Build history of the part. All positions in model axes, mm. Coordinates: 2 decimals unless noted, no trailing zeros. Order: outer loops, then holes, each group sorted by start corner. A loop starts at its lowest first (then second) coordinate and runs counter-clockwise, first axis right, second up. Notation, with made-up numbers: M 12.25,21.5 L 54.25,21.5 A7 ccw 54.25,33.5 Z; hole C 25,25.25 d7. An arc over 180 degrees is marked long. Write item = value, one per line. Start each with the question number.
Q1. Band-saw the part on B-B on x = 95.5. Write the cut outline in (y, z), plus the area to 3 significant figures.
Q2. Band-saw the part on A-A on z = 9.5. Write the cut outline in (x, y).
Q3. Band-saw the part on D-D on x = 34.5. Write the cut outline in (y, z).
Q4. Band-saw the part on C-C on y = -631.5. Write the cut outline in (x, z).
Q5. Drill centre lines: probe 1 along Z at (x, y) = (65, -531); probe 2 along Y at (x, z) = (293, 19.5); probe 3 along Y at (x, z) = (161.5, 29). Where is each one in solid material? Low to high.
Q6. Pin check, flat tips, straight feed: P1, Ø1.1, axis at x = 155, z = -0.5, coming from the +Y side; P2, Ø6, axis at x = 193.5, y = -675, coming from the -Z side; P3, Ø20, axis at x = 293, y = -1080.5, coming from the +Z side; P4, Ø6.5, axis at y = -1114.5, z = 7.5, coming from the +X side. Stop position of each tip, or through.
Q7. Pull direction Z, two halves, no side cores. Call faces 1 (the face through (299, -1083, 20.9)), 2 (the face through (184.49, -576.194, 9.853)), 3 (the face through (162, -606, 41.5)), 4 (the face through (196.1, -567.9, 14.2)): released by +Z, released by -Z, zero draft, split by the parting line, or undercut.
```python
from build123d import *

# Parameters (mm, degrees)
SKETCH_1_W        = 15.2
SKETCH_1_H        = 25
SKETCH_1_W_2      = 15.9
SKETCH_1_W_3      = 60
SKETCH_1_H_2      = 55.8
SKETCH_1_H_3      = 56.6
SKETCH_1_H_4      = 59.4
SKETCH_1_W_4      = 147.9
SKETCH_1_H_5      = 26.5
SKETCH_1_H_6      = 78.6
SKETCH_1_H_7      = 80.6
SKETCH_1_H_8      = 81.1
SKETCH_1_W_5      = 59.5
SKETCH_1_H_9      = 83.5
SKETCH_1_H_10     = 84.1
SKETCH_1_H_11     = 84.6
SKETCH_1_H_12     = 84.7
SKETCH_1_H_13     = 103
SKETCH_1_H_14     = 103.2
SKETCH_1_H_15     = 105.1
SKETCH_1_H_16     = 111.3
SKETCH_1_H_17     = 127.2
SKETCH_1_H_18     = 130
EXTRUDE_1_DEPTH   = 1
SKETCH_2_W        = 45.8
SKETCH_2_H        = 19.3
EXTRUDE_2_DEPTH   = 1
EXTRUDE_3_DEPTH   = 22.9
EXTRUDE_4_DEPTH   = 22.9
SKETCH_6_W        = 0.4
SKETCH_6_H        = 25
EXTRUDE_6_DEPTH   = 40
SKETCH_7_W        = 0.4
SKETCH_7_H        = 25
EXTRUDE_7_DEPTH   = 18
EXTRUDE_720_DEPTH = 22.9


with BuildPart() as part:
    # 草图1 → 拉伸1 (new body)
    with BuildSketch(Plane.XY):
        with Locations((91, -1104.8)):
            Rectangle(SKETCH_1_W, SKETCH_1_H)
        with Locations((106.55, -1104.8)):
            Rectangle(SKETCH_1_W_2, SKETCH_1_H)
        with Locations((113.4, -865.7)):
            Rectangle(SKETCH_1_W_3, SKETCH_1_H_2)
        with Locations((30, -811.2)):
            Rectangle(SKETCH_1_W_3, SKETCH_1_H_3)
        with Locations((30, -306.2)):
            Rectangle(SKETCH_1_W_3, SKETCH_1_H_4)
        with Locations((262.05, -1150.35)):
            Rectangle(SKETCH_1_W_4, SKETCH_1_H_5)
        with Locations((30, -1130.5)):
            Rectangle(SKETCH_1_W_3, SKETCH_1_H_6)
        with Locations((30, -40.3)):
            Rectangle(SKETCH_1_W_3, SKETCH_1_H_7)
        with Locations((113.4, -713.75)):
            Rectangle(SKETCH_1_W_3, SKETCH_1_H_8)
        with Locations((113.15, -421.25)):
            Rectangle(SKETCH_1_W_5, SKETCH_1_H_9)
        with Locations((30, -1049.45)):
            Rectangle(SKETCH_1_W_3, SKETCH_1_H_9)
        with Locations((113.4, -796.05)):
            Rectangle(SKETCH_1_W_3, SKETCH_1_H_9)
        with Locations((30, -965.65)):
            Rectangle(SKETCH_1_W_3, SKETCH_1_H_10)
        with Locations((30, -881.55)):
            Rectangle(SKETCH_1_W_3, SKETCH_1_H_10)
        with Locations((30, -234.2)):
            Rectangle(SKETCH_1_W_3, SKETCH_1_H_11)
        with Locations((30, -378.25)):
            Rectangle(SKETCH_1_W_3, SKETCH_1_H_12)
        with Locations((113.4, -935.95)):
            Rectangle(SKETCH_1_W_3, SKETCH_1_H_12)
        with Locations((113.15, -328)):
            Rectangle(SKETCH_1_W_5, SKETCH_1_H_13)
        with Locations((113.15, -514.6)):
            Rectangle(SKETCH_1_W_5, SKETCH_1_H_14)
        with Locations((30, -730.35)):
            Rectangle(SKETCH_1_W_3, SKETCH_1_H_15)
        with Locations((30, -136.25)):
            Rectangle(SKETCH_1_W_3, SKETCH_1_H_16)
        Polygon((83.4, -978.3), (143.4, -978.3), (143.4, -1092.3), (114.5, -1092.3), (98.6, -1092.3), (83.4, -1092.3), align=None)
        with Locations((30, -614.2)):
            Rectangle(SKETCH_1_W_3, SKETCH_1_H_17)
        with Locations((30, -485.6)):
            Rectangle(SKETCH_1_W_3, SKETCH_1_H_18)
        Polygon((188.1, -1117.3), (188.1, -1092.3), (166.2, -1092.3), (143.4, -1092.3), (114.5, -1092.3), (114.5, -1117.3), (98.6, -1117.3), (83.4, -1117.3), (83.4, -1092.3), (83.4, -978.3), (83.4, -893.6), (83.4, -837.8), (83.4, -754.3), (83.4, -673.2), (143.4, -673.2), (342.5, -673.2), (342.5, -616.2), (192.5, -616.2), (146.7, -616.2), (146.7, -566.2), (142.9, -566.2), (83.4, -566.2), (83.4, -463), (83.4, -379.5), (83.4, -276.5), (83.4, -137.6), (118.4, -137.6), (118.4, -79.7), (83.4, -79.7), (83.4, -23.7), (118.4, -23.7), (118.4, 0), (60, 0), (60, -80.6), (60, -191.9), (60, -276.5), (60, -335.9), (60, -420.6), (60, -550.6), (60, -677.8), (60, -782.9), (60, -839.5), (60, -923.6), (60, -1007.7), (60, -1091.2), (60, -1169.8), (188.1, -1169.8), (188.1, -1163.6), (188.1, -1137.1), align=None)
    extrude(amount=-EXTRUDE_1_DEPTH)

    # 草图2 → 拉伸2 (add)
    with BuildSketch(Plane.XY):
        with Locations((173.2, -606.55)):
            Rectangle(SKETCH_2_W, SKETCH_2_H)
    extrude(amount=-EXTRUDE_2_DEPTH)

    # 草图3 → 拉伸3 (add)
    with BuildSketch(Plane(origin=(173.2, -616.2, 0), x_dir=(0, 0, -1), z_dir=(1, 0, 0))):
        Polygon((-21.04289792, 83.799959106), (-21, 61.3), (-20.5, 61.3), (-20.54289792, 83.799959106), align=None)
        Polygon((-21, 61.3), (0, 19.3), (0.5, 19.3), (-20.5, 61.3), align=None)
    extrude(amount=EXTRUDE_3_DEPTH)

    # 草图4 → 拉伸4 (add)
    with BuildSketch(Plane(origin=(173.2, -616.2, 0), x_dir=(0, 0, -1), z_dir=(1, 0, 0))):
        Polygon((-20.5, 61.3), (-20.5, 83.8), (-21.04289792, 83.799959106), (-21, 61.3), align=None)
    extrude(amount=-EXTRUDE_4_DEPTH)

    # 草图6 → 拉伸6 (add)
    with BuildSketch(Plane(origin=(318, -1163.6, 0), x_dir=(0, 0, -1), z_dir=(1, 0, 0))):
        with Locations((-20.7, 81)):
            Rectangle(SKETCH_6_W, SKETCH_6_H)
        Polygon((-20.9, 68.5), (0.1, 26.5), (0.5, 26.5), (-20.5, 68.5), align=None)
    extrude(amount=-EXTRUDE_6_DEPTH)

    # 草图7 → 拉伸7 (add)
    with BuildSketch(Plane(origin=(318, -1163.6, 0), x_dir=(0, 0, -1), z_dir=(1, 0, 0))):
        with Locations((-20.7, 81)):
            Rectangle(SKETCH_7_W, SKETCH_7_H)
        Polygon((-41.9, 26.5), (-41.5, 26.5), (-20.5, 68.5), (-20.9, 68.5), align=None)
    extrude_7 = extrude(amount=EXTRUDE_7_DEPTH)

    # 镜像1: 拉伸7 across plane
    add(extrude_7.mirror(Plane(origin=(298, -1163.6, 0), x_dir=(0, 0, 1), z_dir=(1, 0, 0))))

    # 草图9 → 凸台-拉伸720 (add)
    with BuildSketch(Plane.ZY.offset(-150.3)):
        Polygon((21, -554.9), (20.5, -554.9), (41.5, -596.9), (41.5, -616.2), (42, -616.2), (42, -596.9), align=None)
    extrude(amount=-EXTRUDE_720_DEPTH)


solid = part.part
```
Recorded:
q1.outline = M -1169.8,-1 L -276.5,-1 L -276.5,0 L -1169.8,0 Z; M -137.6,-1 L -79.7,-1 L -79.7,0 L -137.6,0 Z; M -23.7,-1 L 0,-1 L 0,0 L -23.7,0 Z
q1.area = 975 mm2
q2.outline = M 173.2,-577.9 L 196.1,-577.9 L 196.1,-576.9 L 173.2,-576.9 Z; M 278,-1117.9 L 318,-1117.9 L 318,-1117.1 L 278,-1117.1 Z
q3.outline = M -1169.8,-1 L 0,-1 L 0,0 L -1169.8,0 Z
q4.outline = M 0,-1 L 342.5,-1 L 342.5,0 L 0,0 Z
q5.probe_1 = -1 to 0
q5.probe_2 = -1097.9 to -1097.1
q5.probe_3 = -571.9 to -570.9
q6.P1 = -596.9
q6.P2 = -1
q6.P3 = 20.9
q6.P4 = 318
q7.face_1 = released by +Z
q7.face_2 = released by -Z
q7.face_3 = undercut
q7.face_4 = zero draft
